Geometry check sheet. Reference: the model listing, model coordinates, mm. A direction names the side the tool comes from. Round coordinates to 2 decimals unless told otherwise and drop trailing zeros. Loops run counter-clockwise (first coordinate to the right, second up) from the corner with the lowest first, then second, coordinate; pieces in that order, holes last. Notation, with made-up numbers: M 15,89 L 71,89 A18 ccw 71,104 Z; hole C 62,-20.75 d2. An arc over 180 degrees is marked long. Use one line per item in the form item = value. Start each with the question number.
1. Go/stop test with flat-tipped pins: pin 1 (4 mm diameter, centred on x = -22, z = -2.5, fed in from +Y); pin 2 (5 mm diameter, centred on x = -12.5, z = -4.5, fed in from -Y); pin 3 (11 mm diameter, centred on x = -3.5, y = -6, fed in from -Z); pin 4 (2 mm diameter, centred on x = 15.5, y = -26.65, fed in from -Z). Record where each tip stops, or that it passes through.
2. Set-up check for faces 5 (the cylindrical face through (-5.994, -1.748, 1.183)), 6 (the flat face through (21.3, 0, -3)), 7 (the flat face through (11.1, 13.7, -7.4)): record each of +Z, -Z, +X, -X, +Y, -Y from which the full face is reachable in a straight line by a thin tool's end or side.
3. Cross-section at D-D (y = -13). Record the boundary of the cut face in (x, z).
4. Cross-section at A-A (x = 0). Record the boundary of the cut face in (y, z).
5. Draft check along Z on faces 1 (the cylindrical face through (23.14, -31.4, 2.46)), 2 (the flat face through (-13.9, 13.7, -7.4)), 3 (the flat face through (-2.3, -13.5, 2.4)), 4 (the cylindrical face through (-9.278, 11.976, -5.577)). Enter one of: pulls with the +Z half, pulls with the -Z half, needs draft (parallel to the pull), parting line crosses it, or undercut.
6. Cross-section at C-C (z = 1.5). Record the boundary of the cut face in (x, y), then the cut area to 3 significant figures.
7. Cross-section at B-B (y = 23.3). Record the boundary of the cut face in (x, z).
8. Material ranges on line 1 (X direction, y = 14.1, z = -6); line 2 (Y direction, x = 0, z = 3.5); line 3 (Y direction, x = -15.5, z = 3.6), recorded low to high.
```python
from build123d import *

# Parameters (mm, degrees)
AUFSATZ_LINEAR_AUSTRAGEN1_DEPTH  = 5
SKIZZE2_R                        = 1.75
SKIZZE2_R_2                      = 1.7
SCHNITT_LINEAR_AUSTRAGEN1_DEPTH  = 41.549845869
SKIZZE3_R                        = 11.15
SCHNITT_LINEAR_AUSTRAGEN2_DEPTH  = 2.4
SKIZZE4_R                        = 3
SCHNITT_LINEAR_AUSTRAGEN3_DEPTH  = 41.324310285
SKIZZE9_W                        = 65
SKIZZE9_H                        = 4
AUFSATZ_LINEAR_AUSTRAGEN6_DEPTH  = 12
SKIZZE13_W                       = 8.5
SKIZZE13_H                       = 5
AUFSATZ_LINEAR_AUSTRAGEN8_DEPTH  = 4
AUFSATZ_LINEAR_AUSTRAGEN7_DEPTH  = 2.7
SKIZZE14_R                       = 1.7
SCHNITT_LINEAR_AUSTRAGEN4_DEPTH  = 55.909106713
SKIZZE15_R                       = 3.25
SCHNITT_LINEAR_AUSTRAGEN5_DEPTH  = 3.4
AUFSATZ_LINEAR_AUSTRAGEN9_REACH  = 50.873
AUFSATZ_LINEAR_AUSTRAGEN10_DEPTH = 5
VERRUNDUNG4_R                    = 3
VERRUNDUNG4_OF_SPIEGELN5_R       = 3


with BuildPart() as part:
    # Skizze1 → Aufsatz-Linear austragen1 (new body)
    with BuildSketch(Plane.XY):
        with BuildLine():
            Line((-21, 32.3), (21, 32.3))
            ThreePointArc((21, 32.3), (23.121320344, 31.421320344), (24, 29.3))
            Line((24, 29.3), (24, -29.3))
            ThreePointArc((24, -29.3), (23.121320344, -31.421320344), (21, -32.3))
            Line((21, -32.3), (-21, -32.3))
            ThreePointArc((-21, -32.3), (-23.121320344, -31.421320344), (-24, -29.3))
            Line((-24, -29.3), (-24, 29.3))
            ThreePointArc((-24, 29.3), (-23.121320344, 31.421320344), (-21, 32.3))
        make_face()
    extrude(amount=AUFSATZ_LINEAR_AUSTRAGEN1_DEPTH)

    # Skizze2 → Schnitt-Linear austragen1 (cut, through all)
    with BuildSketch(Plane.XY.offset(5)):
        with Locations((-15.5, -26.65)):
            Circle(SKIZZE2_R)
        with Locations((15.5, -26.65)):
            Circle(SKIZZE2_R)
        with Locations((15.5, 4.35)):
            Circle(SKIZZE2_R)
        with Locations((-15.5, 4.35)):
            Circle(SKIZZE2_R)
        with Locations((-17.5, 23.3)):
            Circle(SKIZZE2_R_2)
        with Locations((17.5, 23.3)):
            Circle(SKIZZE2_R_2)
    extrude(amount=-SCHNITT_LINEAR_AUSTRAGEN1_DEPTH, mode=Mode.SUBTRACT)

    # Skizze3 → Schnitt-Linear austragen2 (cut)
    with BuildSketch(Plane(origin=(0, 0, 0), x_dir=(-1, 0, 0), z_dir=(0, 0, -1))):
        with Locations((0, -11.15)):
            Circle(SKIZZE3_R)
    extrude(amount=-SCHNITT_LINEAR_AUSTRAGEN2_DEPTH, mode=Mode.SUBTRACT)

    # Skizze4 → Schnitt-Linear austragen3 (cut, through all)
    with BuildSketch(Plane(origin=(0, 0, 2.4), x_dir=(-1, 0, 0), z_dir=(0, 0, -1))):
        with Locations((0, -11.15)):
            Circle(SKIZZE4_R)
    extrude(amount=-SCHNITT_LINEAR_AUSTRAGEN3_DEPTH, mode=Mode.SUBTRACT)

    # Skizze9 → Aufsatz-Linear austragen6 (add)
    with BuildSketch(Plane(origin=(0, 0, 0), x_dir=(-1, 0, 0), z_dir=(0, 0, -1))):
        with Locations((0, 12.3)):
            Rectangle(SKIZZE9_W, SKIZZE9_H)
    extrude(amount=AUFSATZ_LINEAR_AUSTRAGEN6_DEPTH)

    # Skizze13 → Aufsatz-Linear austragen8 (add)
    with BuildSketch(Plane(origin=(0, 14.3, 0), x_dir=(1, 0, 0), z_dir=(0, 1, 0))):
        with Locations((28.25, -2.5)):
            Rectangle(SKIZZE13_W, SKIZZE13_H)
    aufsatz_linear_austragen8 = extrude(amount=-AUFSATZ_LINEAR_AUSTRAGEN8_DEPTH)

    # Skizze11 → Aufsatz-Linear austragen7 (add)
    with BuildSketch(Plane(origin=(24, 0, 0), x_dir=(0, 0, -1), z_dir=(1, 0, 0))):
        Polygon((12, 10.3), (0, -29.3), (0, 10.3), align=None)
    aufsatz_linear_austragen7 = extrude(amount=-AUFSATZ_LINEAR_AUSTRAGEN7_DEPTH)

    # Spiegeln4: Aufsatz-Linear austragen8, Aufsatz-Linear austragen7 across plane
    add(aufsatz_linear_austragen8.mirror(Plane.ZY))
    add(aufsatz_linear_austragen7.mirror(Plane.ZY))

    # Skizze14 → Schnitt-Linear austragen4 (cut, through all)
    with BuildSketch(Plane.XZ.offset(-10.3)):
        with Locations(Location((12.5, -6, 0), (0, 0, 270))):
            Circle(SKIZZE14_R)
        with Locations(Location((-12.5, -6, 0), (0, 0, 270))):
            Circle(SKIZZE14_R)
    extrude(amount=-SCHNITT_LINEAR_AUSTRAGEN4_DEPTH, mode=Mode.SUBTRACT)

    # Skizze15 → Schnitt-Linear austragen5 (cut)
    with BuildSketch(Plane(origin=(0, 10.3, 0), x_dir=(-1, 0, 0), z_dir=(0, -1, 0))):
        with Locations(Location((12.5, 6, 0), (0, 0, 90))):
            Circle(SKIZZE15_R)
        with Locations(Location((-12.5, 6, 0), (0, 0, 90))):
            Circle(SKIZZE15_R)
    extrude(amount=-SCHNITT_LINEAR_AUSTRAGEN5_DEPTH, mode=Mode.SUBTRACT)

    # Aufsatz-Linear austragen9: up to this plane
    aufsatz_linear_austragen9_end = Plane(origin=(21.3, 10.3, -12), z_dir=(0, -0.29000739528287084, -0.9570244044334736))
    # Skizze16 → Aufsatz-Linear austragen9 (add, up to the surface)
    with BuildSketch(Plane.XY.offset(5), mode=Mode.PRIVATE) as aufsatz_linear_austragen9_sk1:
        Polygon((32.5, 10.3), (24, -29.3), (24, 10.3), align=None)
    aufsatz_linear_austragen9_tool1 = split(extrude(aufsatz_linear_austragen9_sk1.sketch, amount=-AUFSATZ_LINEAR_AUSTRAGEN9_REACH, mode=Mode.PRIVATE), bisect_by=aufsatz_linear_austragen9_end, keep=Keep.BOTH, mode=Mode.PRIVATE)
    aufsatz_linear_austragen9 = aufsatz_linear_austragen9_tool1.solids().sort_by_distance((26.833333, -2.9, 5))[0]
    add(aufsatz_linear_austragen9)

    # Skizze17 → Aufsatz-Linear austragen10 (add)
    with BuildSketch(Plane.XY.offset(5)):
        Polygon((21, 32.3), (32.5, 32.3), (32.5, 14.3), (24, 14.3), align=None)
    aufsatz_linear_austragen10 = extrude(amount=-AUFSATZ_LINEAR_AUSTRAGEN10_DEPTH)

    # Verrundung4
    verrundung4_edges = [part.edges().sort_by_distance(p)[0] for p in [
        (32.5, 32.3, 2.5),
    ]]
    fillet(verrundung4_edges, radius=VERRUNDUNG4_R)

    # Spiegeln5: Aufsatz-Linear austragen9, Aufsatz-Linear austragen10 across plane
    add(aufsatz_linear_austragen9.mirror(Plane.ZY))
    add(aufsatz_linear_austragen10.mirror(Plane.ZY))

    # Verrundung4 of Spiegeln5
    verrundung4_of_spiegeln5_edges = [part.edges().sort_by_distance(p)[0] for p in [
        (-32.5, 32.3, 2.5),
    ]]
    fillet(verrundung4_of_spiegeln5_edges, radius=VERRUNDUNG4_OF_SPIEGELN5_R)


solid = part.part
```
Reported:
q1.pin_1 = 14.3
q1.pin_2 = 10.3
q1.pin_3 = 0
q1.pin_4 = through
q2.face_5 = -Z
q2.face_6 = -Z, -Y
q2.face_7 = -Y
q3.outline = M -27.5,-4.94 L -21.3,-4.94 L -21.3,0 L -11,0 L -11,2.4 L -2.36,2.4 L -2.36,5 L -27.5,5 Z; M 2.36,2.4 L 11,2.4 L 11,0 L 21.3,0 L 21.3,-4.94 L 27.5,-4.94 L 27.5,5 L 2.36,5 Z
q4.outline = M -32.3,0 L -22.3,0 L -22.3,2.4 L -14.15,2.4 L -14.15,5 L -32.3,5 Z; M -8.15,2.4 L 0,2.4 L 0,0 L 10.3,0 L 10.3,-12 L 14.3,-12 L 14.3,0 L 32.3,0 L 32.3,5 L -8.15,5 Z
q5.face_1 = needs draft
q5.face_2 = undercut
q5.face_3 = pulls with the -Z half
q5.face_4 = undercut
q6.outline = M -32.5,10.3 L -24,-29.3 A3 ccw -21,-32.3 L 21,-32.3 A3 ccw 24,-29.3 L 32.5,10.3 L 32.5,29.3 A3 ccw 29.5,32.3 L -29.5,32.3 A3 ccw -32.5,29.3 Z; hole C -17.5,23.3 d3.4; hole C -15.5,-26.65 d3.5; hole C -15.5,4.35 d3.5; hole C 0,-11.15 d22.3; hole C 15.5,-26.65 d3.5; hole C 15.5,4.35 d3.5; hole C 17.5,23.3 d3.4
q6.area = 3,360 mm²
q7.outline = M -32.5,0 L -19.2,0 L -19.2,5 L -32.5,5 Z; M -15.8,0 L 15.8,0 L 15.8,5 L -15.8,5 Z; M 19.2,0 L 32.5,0 L 32.5,5 L 19.2,5 Z
q8.line_1 = -32.5 to -14.2, -10.8 to 10.8, 14.2 to 32.5
q8.line_2 = -32.3 to -14.15, -8.15 to 32.3
q8.line_3 = -32.3 to -28.4, -24.9 to 2.6, 6.1 to 32.3
